Build history of the part. All positions in model axes, mm. Give positions to 0.01 mm unless a question says otherwise; leave off trailing zeros. Order: outer loops, then holes, each group sorted by start corner. A loop starts at its lowest first (then second) coordinate and runs counter-clockwise, first axis right, second up. Notation, with made-up numbers: (-1.75, 22) - (4.25, 22) arc R20 ccw to (4.25, 39) - close; hole circle Ø8 at (-21, 40.5). An arc over 180 degrees is marked (long way). Write each question's results on one line, items separated by ' | '. Start each with the question number.
1) Cut at A-A on x = 0. List the corners of the cut face in (y, z).
2) Cut at C-C on z = 49. List the corners of the cut face in (x, y).
3) Cut at D-D on x = 46.5. List the corners of the cut face in (y, z), plus the area to 3 significant figures.
4) Drill centre lines: line 1 along X through (y, z) = (19.25, 0); line 2 along Z through (x, y) = (21.5, 6.75); line 3 along X through (y, z) = (16.5, -44). Where is each one in solid material? Low to high. Write a range as from..to.
5) Cut at B-B on y = 10.5. List the corners of the cut face in (x, z), plus the area to 3 significant figures.
6) Drop flat-ended pins along their axis: pin 1 Ø6 at (x, z) = (22.59, 4.31) entering from +Y; pin 2 Ø8 at (y, z) = (6, -53) entering from +X; pin 3 Ø3 at (y, z) = (9, 52) entering from -X; pin 4 Ø8 at (y, z) = (21, -32.5) entering from -X. Give the stop position or say it passes through.
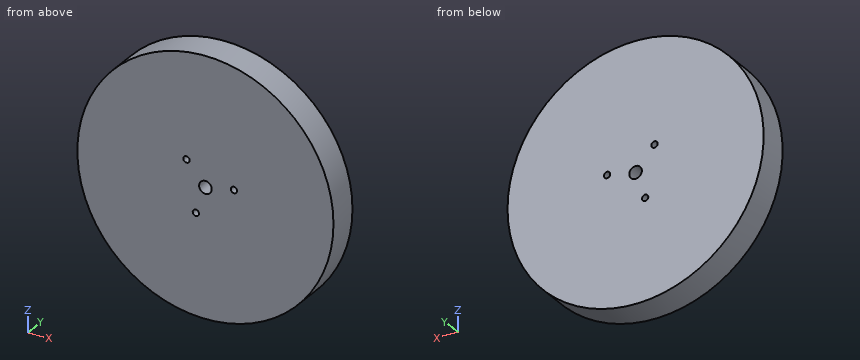
from build123d import *

# Parameters (mm, degrees)
SKETCH1_R           = 101.6
SKETCH1_R_2         = 5
BOSS_EXTRUDE8_DEPTH = 25
SKETCH2_R           = 2.5
CUT_EXTRUDE1_DEPTH  = 26


with BuildPart() as part:
    # Sketch1 → Boss-Extrude8 (new body)
    with BuildSketch(Plane(origin=(0, 0, 0), x_dir=(1, 0, 0), z_dir=(0, 1, 0))):
        Circle(SKETCH1_R)
        Circle(SKETCH1_R_2, mode=Mode.SUBTRACT)
    extrude(amount=BOSS_EXTRUDE8_DEPTH)

    # Sketch2 → Cut-Extrude1 (cut, through all)
    with BuildSketch(Plane.XZ):
        with Locations((22.59307321, 4.307324334)):
            Circle(SKETCH2_R)
        with Locations((-7.56628431, -21.719837517)):
            Circle(SKETCH2_R)
        with Locations((-15.026788901, 17.412513183)):
            Circle(SKETCH2_R)
    extrude(amount=-CUT_EXTRUDE1_DEPTH, mode=Mode.SUBTRACT)


solid = part.part
Results:
1) outline: (0, -101.6) - (25, -101.6) - (25, -5) - (0, -5) - close; (0, 5) - (25, 5) - (25, 101.6) - (0, 101.6) - close
2) outline: (-89, 0) - (89, 0) - (89, 25) - (-89, 25) - close
3) outline: (0, -90.33) - (25, -90.33) - (25, 90.33) - (0, 90.33) - close | area: 4,520 mm^2
4) line 1: -101.6..-5, 5..101.6 | line 2: -99.3..2.06, 6.56..99.3 | line 3: -91.58..91.58
5) outline: circle Ø203.2 at (0, 0); hole circle Ø5 at (-15.03, 17.41); hole circle Ø5 at (-7.57, -21.72); hole circle Ø10 at (0, 0); hole circle Ø5 at (22.59, 4.31) | area: 32,300 mm^2
6) pin 1: y = 25 | pin 2: x = 89 | pin 3: x = -88.16 | pin 4: x = -97.52
